Check sheet for the modelled part. Datum: model origin and axes. Units: mm. A direction names the side the tool comes from. Round coordinates to 2 decimals unless told otherwise and drop trailing zeros. Loops run counter-clockwise (first coordinate to the right, second up) from the corner with the lowest first, then second, coordinate; pieces in that order, holes last. Notation, with made-up numbers: (52, 2) -> (57, 2) arc R24 cw to (57, 26) -> close; hole circle Ø6 at (26, 77). An arc over 180 degrees is marked (long way). One line per item, written item: value. Start each with the question number.
1. Material ranges on L1, parallel to Y at x = -16.5, z = -36; L2, parallel to X at y = 14.5, z = -10; L3, parallel to Z at x = -17.5, y = 2, recorded low to high.
2. Go/stop test with flat-tipped pins: pin 1 (2 mm diameter, centred on y = 7, z = -36, fed in from +X); pin 2 (4 mm diameter, centred on x = -46, y = 12, fed in from +Z); pin 3 (10 mm diameter, centred on x = -21, z = -33.5, fed in from +Y). Record where each tip stops, or that it passes through.
3. Cross-section at B-B on y = 15. Record the cut outline in (x, z).
4. Release check for a two-part mould opening along X. For faces 3 (the face through (0.55, 18.96, -12.61)), 4 (the face through (-13, 38.1, -2)), 5 (the face through (13.601, 25.222, -7.074)), 6 (the face through (8.59, 9.48, -9.37)) record: +X half, -X half, draft (parallel to the pull), parting line (faces both ways), or undercut.
5. Set-up check for faces 1 (the face through (-11, 6.35, 11)), 2 (the face through (-11, 12.7, -12)): record each of +Z, -Z, +X, -X, +Y, -Y from which the full face is reachable in a straight line by a thin tool's end or side.
from build123d import *

# Parameters (mm, degrees)
SKETCH1_R           = 63.475313381
BOSS_EXTRUDE1_DEPTH = 12.7
FILLET2_R           = 12.7
SHELL2_T            = -6.35
SKETCH2_R           = 12.710048884
CUT_EXTRUDE1_DEPTH  = 12.7
SKETCH4_R           = 15.331222423
BOSS_EXTRUDE2_DEPTH = 25.4
SKETCH5_R           = 12.620209495
CUT_EXTRUDE2_DEPTH  = 27.94
SKETCH11_R          = 12.723642388
CUT_EXTRUDE4_DEPTH  = 12.7


with BuildPart() as part:
    # Sketch1 → Boss-Extrude1 (new body)
    with BuildSketch(Plane(origin=(0, 0, 0), x_dir=(1, 0, 0), z_dir=(0, 1, 0))):
        with Locations(Location((0, 0, 0), (0, 0, 270))):
            Circle(SKETCH1_R)
    extrude(amount=BOSS_EXTRUDE1_DEPTH)

    # Fillet2
    fillet2_edges = [part.edges().sort_by_distance(p)[0] for p in [
        (0, 12.7, -63.475313381),
    ]]
    fillet(fillet2_edges, radius=FILLET2_R - 0.0001)  # a hair under: the kernel refuses the full size

    # Shell2
    shell2_openings = [part.faces().sort_by_distance(p)[0] for p in [
        (0, 0, 0),
    ]]
    offset(amount=SHELL2_T, openings=shell2_openings)

    # Sketch2 → Cut-Extrude1 (cut)
    with BuildSketch(Plane(origin=(0, 0, 0), x_dir=(1, 0, 0), z_dir=(0, 1, 0))):
        with Locations(Location((0, 0, 0), (0, 0, 270))):
            Circle(SKETCH2_R)
    extrude(amount=CUT_EXTRUDE1_DEPTH, mode=Mode.SUBTRACT)

    # Sketch4 → Boss-Extrude2 (add)
    with BuildSketch(Plane(origin=(0, 12.7, 0), x_dir=(1, 0, 0), z_dir=(0, 1, 0))):
        with Locations(Location((0, 0, 0), (0, 0, 90))):
            Circle(SKETCH4_R)
    extrude(amount=BOSS_EXTRUDE2_DEPTH)

    # Sketch5 → Cut-Extrude2 (cut)
    with BuildSketch(Plane(origin=(0, 0, 0), x_dir=(1, 0, 0), z_dir=(0, 1, 0))):
        with Locations(Location((0, 0, 0), (0, 0, 270))):
            Circle(SKETCH5_R)
    extrude(amount=CUT_EXTRUDE2_DEPTH, mode=Mode.SUBTRACT)

    # Sketch11 → Cut-Extrude4 (cut)
    with BuildSketch(Plane(origin=(0, 38.1, 0), x_dir=(1, 0, 0), z_dir=(0, 1, 0))):
        with Locations(Location((0, 0, 0), (0, 0, 270))):
            Circle(SKETCH11_R)
    extrude(amount=-CUT_EXTRUDE4_DEPTH, mode=Mode.SUBTRACT)


solid = part.part
Taken from the geometry:
1. L1: y = 6.35 to 12.7
1. L2: x = -11.62 to -7.7, 7.7 to 11.62
1. L3: z = -60.85 to -54.04, 54.04 to 60.85
2. pin 1: stops at x = 50.74
2. pin 2: stops at z = 36.99
2. pin 3: stops at y = 12.7
3. outline: circle Ø30.66 at (0, 0); hole circle Ø25.24 at (0, 0)
4. face 3: undercut
4. face 4: draft
4. face 5: parting line
4. face 6: undercut
5. face 1: -Y
5. face 2: +Y
